Can you work these out from the model? Positions are in its coordinate system, mm. Face numbers are marked on the shaded views. A direction names the side the tool comes from. Give positions to 0.01 mm unless a question says otherwise; leave off trailing zeros. Order: outer loops, then holes, each group sorted by start corner. A loop starts at its lowest first (then second) coordinate and runs counter-clockwise, first axis right, second up. Notation, with made-up numbers: M -15.5,23 L 4.5,23 A27 ccw 4.5,56 Z; hole C 13,70 d5. An arc over 180 degrees is marked long. Use a Markdown table: item, result. Add a question column.
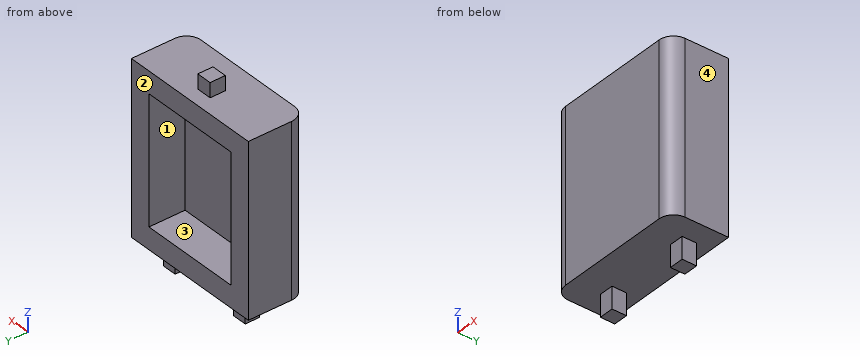
from build123d import *

# Parameters (mm, degrees)
SKETCH1_W                = 2.1
SKETCH1_H                = 2.1
BOSS_EXTRUDE1_DEPTH      = 2
SKETCH4_W                = 2.2
SKETCH4_H                = 2.2
BOSS_EXTRUDE3_DEPTH      = 2
SWEEP4_START             = -1.1
SWEEP4_DEPTH             = 2.2
SKETCH8_W                = 2.2
SKETCH8_H                = 2.2
SKETCH8_W_2              = 2
SKETCH8_H_2              = 2
CUT_EXTRUDE2_DEPTH       = 5
SKETCH9_W                = 2
SKETCH9_H                = 2
CUT_EXTRUDE3_DEPTH       = 2
BOSS_EXTRUDE4_DEPTH      = 3
BOSS_EXTRUDE4_DEPTH_BACK = 5
SKETCH10_W               = 20
SKETCH10_H               = 23.5
SKETCH11_W               = 14
SKETCH11_H               = 17.5
CUT_EXTRUDE4_DEPTH       = 5
FILLET1_R                = 2


# Read off the part's stored shape, not the designer's step: Sweep4
with BuildPart() as part:
    # Sketch1 → Boss-Extrude1 (new body)
    with BuildSketch(Plane.XY):
        Rectangle(SKETCH1_W, SKETCH1_H)
    extrude(amount=BOSS_EXTRUDE1_DEPTH)

    # Sketch4 → Boss-Extrude3 (add)
    with BuildSketch(Plane.XY):
        Rectangle(SKETCH4_W, SKETCH4_H)
    extrude(amount=-BOSS_EXTRUDE3_DEPTH)

    # Sweep4 outline → Sweep4 (add)
    with BuildSketch(Plane(origin=(0, 0, 0), x_dir=(1, 0, 0), z_dir=(0, 1, 0)).offset(SWEEP4_START)):
        with BuildLine():
            Line((7.09999865, 11.165148445), (7.09999919, 28.5))
            Line((7.09999919, 28.5), (4.89999919, 28.5))
            Line((4.89999919, 28.5), (4.89999865, 11.165148445))
            ThreePointArc((4.89999865, 11.165148445), (4.099633159, 8.481308894), (1.959999989, 6.674225732))
            ThreePointArc((1.959999989, 6.674225732), (-0.2669663, 4.793384792), (-1.1, 2))
            Line((-1.1, 2), (1.1, 2))
            ThreePointArc((1.1, 2), (1.573685829, 3.588395274), (2.839999687, 4.657893766))
            ThreePointArc((2.839999687, 4.657893766), (5.940285288, 7.276319376), (7.09999865, 11.165148445))
        make_face()
    sweep4 = extrude(amount=SWEEP4_DEPTH)

    # Mirror1: Sweep4 across plane
    add(sweep4.mirror(Plane(origin=(0, 0, 0), x_dir=(0, 0, 1), z_dir=(1, 0, 0))))

    # Sketch8 → Cut-Extrude2 (cut)
    with BuildSketch(Plane(origin=(0, 0, -28.5), x_dir=(-1, 0, 0), z_dir=(0, 0, -1))):
        with Locations((-5.99999919, 0)):
            Rectangle(SKETCH8_W, SKETCH8_H)
        with Locations((-5.99999919, 0)):
            Rectangle(SKETCH8_W_2, SKETCH8_H_2, mode=Mode.SUBTRACT)
    cut_extrude2 = extrude(amount=-CUT_EXTRUDE2_DEPTH, mode=Mode.SUBTRACT)

    # Sketch9 → Cut-Extrude3 (cut)
    with BuildSketch(Plane(origin=(0, 0, -28.5), x_dir=(-1, 0, 0), z_dir=(0, 0, -1))):
        with Locations((-5.99999919, 0)):
            Rectangle(SKETCH9_W, SKETCH9_H)
    cut_extrude3 = extrude(amount=-CUT_EXTRUDE3_DEPTH, mode=Mode.SUBTRACT)

    # Mirror2: Cut-Extrude2, Cut-Extrude3 across plane
    add(cut_extrude2.mirror(Plane(origin=(0, 0, 0), x_dir=(0, 0, 1), z_dir=(1, 0, 0))), mode=Mode.SUBTRACT)
    add(cut_extrude3.mirror(Plane(origin=(0, 0, 0), x_dir=(0, 0, 1), z_dir=(1, 0, 0))), mode=Mode.SUBTRACT)

    # Sketch10 → Boss-Extrude4 (add, two sides: drawn at the far end of the back side and taken through both)
    with BuildSketch(Plane(origin=(0, 0, 0), x_dir=(1, 0, 0), z_dir=(0, 1, 0)).offset(-BOSS_EXTRUDE4_DEPTH_BACK)):
        with Locations((0, 11.75)):
            Rectangle(SKETCH10_W, SKETCH10_H)
    extrude(amount=BOSS_EXTRUDE4_DEPTH + BOSS_EXTRUDE4_DEPTH_BACK)

    # Sketch11 → Cut-Extrude4 (cut)
    with BuildSketch(Plane(origin=(0, 3, 0), x_dir=(1, 0, 0), z_dir=(0, 1, 0))):
        with Locations((0, 11.75)):
            Rectangle(SKETCH11_W, SKETCH11_H)
    extrude(amount=-CUT_EXTRUDE4_DEPTH, mode=Mode.SUBTRACT)

    # Fillet1
    fillet1_edges = [part.edges().sort_by_distance(p)[0] for p in [
        (-10, -5, -11.75),
        (10, -5, -11.75),
    ]]
    fillet(fillet1_edges, radius=FILLET1_R)


solid = part.part
1. If we section it at D-D, the plane y = -0.5: List the corners of the cut face in (x, z) for me, then the cut area to 3 significant figures.
2. If we section it at A-A, the plane y = 2.25: List the corners of the cut face in (x, z) for me, then the cut area to 3 significant figures.
3. Will these pins go through, and if not, where does the flat tip stop? pin 1 (1.6 mm diameter, centred on y = 0, z = 1.5, fed in from +X); pin 2 (2 mm diameter, centred on x = -4, z = -9, fed in from +Y); pin 3 (3 mm diameter, centred on x = 4, y = -4, fed in from -Z).
4. We'd pull the mould along Z, two halves only. Please class the marked faces 1 and 2: +Z half, -Z half, draft (parallel to the pull), parting line (faces both ways), or undercut.
5. If we section it at B-B, the plane z = -7: List the corners of the cut face in (x, y) for me.
6. On a 3-axis mill with a long thin cutter (end or side, diameter ignored), from which of +Z, -Z, +X, -X, +Y, -Y can I reach the whole of each face in a straight line? I mean the marked faces 3 and 4. Say none if no direction works.
7. If we section it at C-C, the plane x = 6.25: List the corners of the cut face in (y, z) for me, then the cut area to 4 significant figures.
8. I need wall thicknesses on L1, parallel to X at y = -0.75, z = -16; L2, parallel to Z at x = 1, y = -0.25; L3, parallel to Z at x = -4, y = -0.5. Which ranges of each line are inside material? Lowest first, please. Write a range as [from, to].
Geometry results:
| question | item | result |
|---|---|---|
| 1 | outline | M -10,-23.5 L -7,-23.5 L -7,-26.5 L -5,-26.5 L -5,-23.5 L 5,-23.5 L 5,-26.5 L 7,-26.5 L 7,-23.5 L 10,-23.5 L 10,0 L 1.05,0 L 1.05,2 L -1.05,2 L -1.05,0 L -10,0 Z; hole M -7,-20.5 L 7,-20.5 L 7,-3 L -7,-3 Z |
| 1 | area | 241 mm^2 |
| 2 | outline | M -10,-23.5 L 10,-23.5 L 10,0 L -10,0 Z; hole M -7,-20.5 L 7,-20.5 L 7,-3 L -7,-3 Z |
| 2 | area | 225 mm^2 |
| 3 | pin 1 | stops at x = 1.05 |
| 3 | pin 2 | stops at y = -2 |
| 3 | pin 3 | stops at z = -23.5 |
| 4 | face 1 | undercut |
| 4 | face 2 | draft |
| 5 | outline | M -10,-3 A2 ccw -8,-5 L 8,-5 A2 ccw 10,-3 L 10,3 L 7,3 L 7,-2 L -7,-2 L -7,3 L -10,3 Z |
| 6 | face 3 | +Y |
| 6 | face 4 | +Z, -Z, +X, +Y, -Y |
| 7 | outline | M -5,-23.5 L -1,-23.5 L -1,-26.5 L 1,-26.5 L 1,-23.5 L 3,-23.5 L 3,-20.5 L -2,-20.5 L -2,-3 L 3,-3 L 3,0 L -5,0 Z |
| 7 | area | 106.5 mm^2 |
| 8 | L1 | x = [-10, -7], [7, 10] |
| 8 | L2 | z = [-23.5, -20.5], [-3, 2] |
| 8 | L3 | z = [-23.5, -20.5], [-3, 0] |
